Source: CAD feature listing. Evaluate the final solid. Frame: model axes, mm. A direction names the side the tool comes from. Give positions to 0.01 mm unless a question says otherwise; leave off trailing zeros. Loops run counter-clockwise (first coordinate to the right, second up) from the corner with the lowest first, then second, coordinate; pieces in that order, holes last. Notation, with made-up numbers: (-30.5, 27.5) - (-25.5, 27.5) arc R11 ccw to (-25.5, 46.5) - close; hole circle Ø4 at (56.25, 74.5). An arc over 180 degrees is marked (long way). Write each question's results on one line, items separated by ' | '. Start each with the question number.
(1) Reachability of faces 1 (the flat face through (25.9, -8, -11)), 2 (the flat face through (-19, -8, 4)), 3 (the flat face through (19, -8, 4)) from +Z, -Z, +X, -X, +Y, -Y: full face, straight path, thin tool, end or side. Return the list, or none.
(2) Cut plane B-B on y = -8.75. Return the cut outline in (x, z), then the cut area to 3 significant figures.
(3) Cut plane D-D on z = 7. Return the cut outline in (x, y).
(4) Contact query for flat-ended pins moving along their axis: pin 1 (2 mm diameter, centred on x = -19, y = -4.5, fed in from +Z); pin 2 (3 mm diameter, centred on y = -8.5, z = 7, fed in from -X). Output: stop coordinate, or through.
(5) Pull-direction query (X, two-part tool) for faces 4 (the flat face through (29.9, -8, -8)), 5 (the flat face through (0, 0, 1)), 6 (the cylindrical face through (-25.91, -8.01, 0.08)); classes: pulls with the +X half, pulls with the -X half, needs draft (parallel to the pull), parting line crosses it, or undercut.
(6) Cut plane A-A on z = -10.75. Return the cut outline in (x, y).
(7) Cut plane C-C on x = 5. Return the cut outline in (y, z).
(8) Material intervals for line 1 along X through (y, z) = (-5.25, -4.5); line 2 along X through (y, z) = (-3.5, -1.5); line 3 along Z through (x, y) = (-24.5, -14.5), sorted ascending. Write a range as [from, to].
from build123d import *

# Parameters (mm, degrees)
F1_DEPTH = 15.8
F2_W     = 15
F2_H     = 15.8
F3_DEPTH = 5.5
F4_R     = 2
F5_DEPTH = 15.801


with BuildPart() as f1:
    # F0 (on Front) → F1 (new body)
    with BuildSketch(Plane.XZ):
        Polygon((-25.9, -20), (-25.9, 0), (25.9, 0), (25.9, -20), (29.9, -20), (29.9, 4), (-29.9, 4), (-29.9, -20), align=None)
    extrude(amount=F1_DEPTH)

    # F2 (on face) → F3 (join)
    with BuildSketch(Plane.XY.offset(4)):
        with Locations((0, -7.9)):
            Rectangle(F2_W, F2_H)
    extrude(amount=F3_DEPTH)

    # F4 (on face) → F5 (cut, through all)
    with BuildSketch(Plane.XZ.offset(15.8)):
        with Locations((-24.52996, -1.37004)):
            Circle(F4_R)
        with Locations((24.52996, -1.37004)):
            Circle(F4_R)
    extrude(amount=-F5_DEPTH, mode=Mode.SUBTRACT)


solid = f1.part
Ans:
1) face 1: -Z, +Y, -Y | face 2: +Z, -X, +Y, -Y | face 3: +Z, +X, +Y, -Y
2) outline: (-29.9, -20) - (-25.9, -20) - (-25.9, -2.83) arc R2 cw (long way) to (-23.07, 0) - (23.07, 0) arc R2 cw (long way) to (25.9, -2.83) - (25.9, -20) - (29.9, -20) - (29.9, 4) - (7.5, 4) - (7.5, 9.5) - (-7.5, 9.5) - (-7.5, 4) - (-29.9, 4) - close | area: 477 mm^2
3) outline: (-7.5, -15.8) - (7.5, -15.8) - (7.5, 0) - (-7.5, 0) - close
4) pin 1: z = 4 | pin 2: x = -7.5
5) face 4: pulls with the +X half | face 5: needs draft | face 6: undercut
6) outline: (-29.9, -15.8) - (-25.9, -15.8) - (-25.9, 0) - (-29.9, 0) - close; (25.9, -15.8) - (29.9, -15.8) - (29.9, 0) - (25.9, 0) - close
7) outline: (-15.8, 0) - (0, 0) - (0, 9.5) - (-15.8, 9.5) - close
8) line 1: [-29.9, -25.9], [25.9, 29.9] | line 2: [-29.9, -26.53], [26.53, 29.9] | line 3: [0.63, 4]
